Geometry check sheet. Reference: the model listing, model coordinates, mm. Face numbers are marked on the shaded views. A direction names the side the tool comes from. Give positions to 0.01 mm unless a question says otherwise; leave off trailing zeros. Use a Markdown table: item, result. Add a question column.
1. Depth check by flat-ended pin: P1, Ø4, axis at x = 3, y = 6.5, coming from the +Z side; P2, Ø1.5, axis at x = 2.5, y = 6.5, coming from the -Z side; P3, Ø1.5, axis at x = -2, y = 2, coming from the -Z side. Enter the tip coordinate at first touch or a pass-through.
2. Material ranges on L1, parallel to Y at x = -3, z = -5.5; L2, parallel to X at y = 4, z = 0; L3, parallel to X at y = 2.75, z = 0, recorded low to high.
3. Draft check along X on the marked faces 3, 4, 5 and 6. Enter one of: pulls with the +X half, pulls with the -X half, needs draft (parallel to the pull), parting line crosses it, or undercut.
4. Set-up check for the marked faces 1 and 2: record each of +Z, -Z, +X, -X, +Y, -Y from which the full face is reachable in a straight line by a thin tool's end or side.
Autodesk Inventor part; units mm, degrees
ref_plane "YZ Plane" through (0, 0, 0) normal (1, 0, 0) x (0, 1, 0)
ref_plane "XZ Plane" through (0, 0, 0) normal (0, 1, 0) x (-1, 0, 0)
ref_plane "XY Plane" through (0, 0, 0) normal (0, 0, 1) x (1, 0, 0)
sketch "Sketch1" plane through (0, 0, 0) normal (0, 1, 0) x (-1, 0, 0)
  circle A0 centre (0, 0) radius 7
  circle A1 centre (0, 0) radius 2.1
  dimension "d0" = 14
  dimension "d1" = 4.2
extrude "Extrusion1" add sketch "Sketch1" along normal blind 2.5
sketch "Sketch2" plane through (0, 2.5, 0) normal (0, 1, 0) x (1, 0, 0)
  circle A0 centre (0, 0) radius 2.1
  line L0 (4.7343, 0) -> (2.3671, -4.1)
  line L1 (2.3671, -4.1) -> (-2.3671, -4.1)
  line L2 (-2.3671, -4.1) -> (-4.7343, 0)
  line L3 (-4.7343, 0) -> (-2.3671, 4.1)
  line L4 (-2.3671, 4.1) -> (2.3671, 4.1)
  line L5 (2.3671, 4.1) -> (4.7343, 0)
  dimension "d10" = 2
  dimension "d11" = 4.2
extrude "Extrusion2" add sketch "Sketch2" along normal blind 6
chamfer "Chamfer1" distance 0.25 angle 45 3 edges at (7, 0, 0) (-2.1, 8.5, 0) (2.1, 0, 0)
draft "FaceDraft1" angle 4 pull direction (0, 1, 0) faces at (3.1562, 4.5, 2.7333) (-0.789, 4.5, 4.1) (3.9452, 4.5, -1.3667) (-3.9452, 4.5, 1.3667) (-3.1562, 4.5, -2.7333) (0.789, 4.5, -4.1) fixed edges at (3.5507, 2.5, 2.05) (0, 2.5, 4.1) (3.5507, 2.5, -2.05) (-3.5507, 2.5, 2.05) (-3.5507, 2.5, -2.05) (0, 2.5, -4.1)
fillet "Fillet1" radius 0.5 6 edges at (2.246, 5.5, -3.8902) (-2.246, 5.5, 3.8902) (2.246, 5.5, 3.8902) (-2.246, 5.5, -3.8902) (4.492, 5.5, 0) (-4.492, 5.5, 0)
properties part number "TeflonHolderWasher"
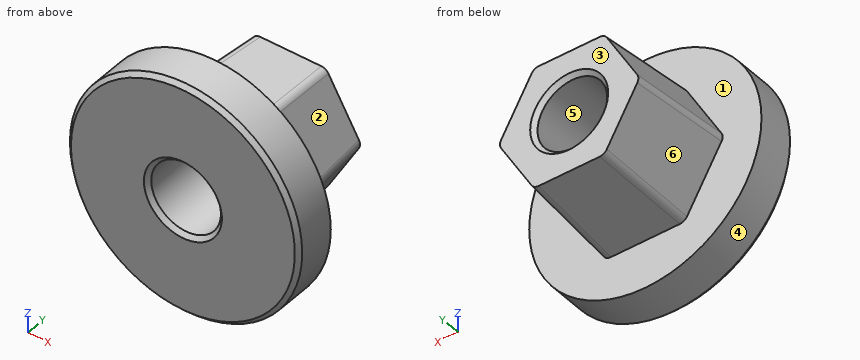
Values found:
| question | item | result |
|---|---|---|
| 1 | P1 | stops at z = 3.94 |
| 1 | P2 | stops at z = -3.86 |
| 1 | P3 | stops at z = -6.89 |
| 2 | L1 | y = 0 to 2.5 |
| 2 | L2 | x = -4.54 to -2.1, 2.1 to 4.54 |
| 2 | L3 | x = -4.64 to -2.1, 2.1 to 4.64 |
| 3 | face 3 | needs draft |
| 3 | face 4 | parting line crosses it |
| 3 | face 5 | undercut |
| 3 | face 6 | pulls with the -X half |
| 4 | face 1 | +Y |
| 4 | face 2 | +Z, +X, +Y |
